```python
from build123d import *

# Parameters (mm, degrees)
F0_W     = 60
F0_H     = 20.115981
F0_R     = 3
F0_R_2   = 1.308767
F1_DEPTH = 10
F3_R     = 6
F4_W     = 7.989561
F4_H     = 2.429715
F5_DEPTH = 10


with BuildPart() as f1:
    # F0 (on Front) → F1 (new body)
    with BuildSketch(Plane.XZ):
        with Locations((30, 10.05799)):
            Rectangle(F0_W, F0_H)
        with Locations((6.314433, 11.456186)):
            Circle(F0_R, mode=Mode.SUBTRACT)
        with Locations((26.120204, 12.682377)):
            Circle(F0_R_2, mode=Mode.SUBTRACT)
        with Locations((50, 11.406668)):
            Circle(F0_R, mode=Mode.SUBTRACT)
    extrude(amount=F1_DEPTH)

    # F3
    f3_edges = [f1.edges().sort_by_distance(p)[0] for p in [
        (0, -5, 0),
        (0, -5, 20.115981),
        (60, -5, 0),
        (60, -5, 20.115981),
    ]]
    fillet(f3_edges, radius=F3_R)

    # F4 (on face) → F5 (cut)
    with BuildSketch(Plane.XY.offset(20.115981)):
        with Locations((24.271051, -1.214857)):
            Rectangle(F4_W, F4_H)
    extrude(amount=-F5_DEPTH, mode=Mode.SUBTRACT)


solid = f1.part
```
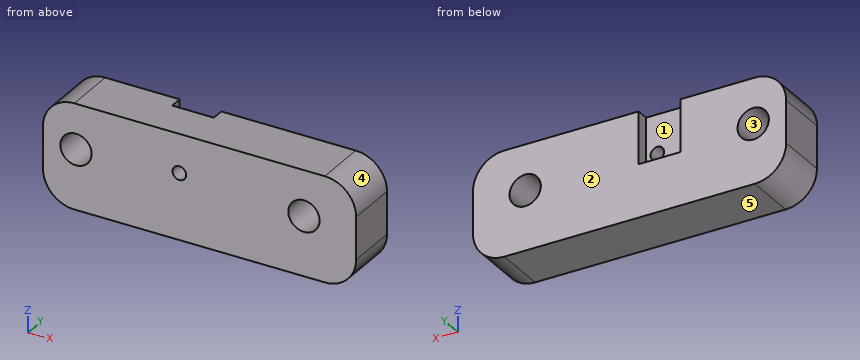
Model file for the job. Use its own axes, mm. Face numbers are marked on the shaded views. A direction names the side the tool comes from. Give positions to 0.01 mm unless a question says otherwise; leave off trailing zeros. Loops run counter-clockwise (first coordinate to the right, second up) from the corner with the lowest first, then second, coordinate; pieces in that order, holes last. Notation, with made-up numbers: (1.25, -13.5) -> (13.25, -13.5) arc R19 ccw to (13.25, 13.5) -> close; hole circle Ø9 at (28.5, 83). An arc over 180 degrees is marked (long way). Use CSV: the item, a comma, the result in double quotes. Start each with the question number.
1) Wall check: line 1 (Z direction, x = 50, y = -6.5); line 2 (X direction, y = -0.75, z = 9); line 3 (X direction, y = -6.25, z = 9.75). Give the ranges that are in metal, low to high.
2) Flat gauge pins, fed straight in: pin 1 Ø4 at (x, z) = (25.5, 15) entering from +Y; pin 2 Ø5.5 at (x, z) = (50, 11.41) entering from -Y; pin 3 Ø2.5 at (x, y) = (22.5, -0.5) entering from +Z; pin 4 Ø0.7 at (y, z) = (-1.5, 15.5) entering from +X. Where does each tip first touch, or does it go through?
3) Slice it at C-C on z = 18.5. Give the cut face in (x, y), plus the area to 3 significant figures.
4) Mould opens along X. For the marked faces 3, 4 and 5 say: released by +X, released by -X, zero draft, split by the parting line, or undercut.
5) Tool access for the marked faces 1 and 2: list every direction of +Z, -Z, +X, -X, +Y, -Y with a clear straight run to the whole face (end or side of a thin tool).
6) Slice it at B-B on y = -0.75. Give the cut face in (x, z).
7) Slice it at A-A on x = 50. Give the cut face in (y, z).
8) Slice it at D-D on y = -8. Give the cut face in (x, z).
Computed values:
1,line 1,"z = 0 to 8.41, 14.41 to 20.12"
1,line 2,"x = 0 to 4.59, 8.04 to 48.21, 51.79 to 60"
1,line 3,"x = 0 to 3.85, 8.78 to 47.5, 52.5 to 60"
2,pin 1,"stops at y = -2.43"
2,pin 2,"passes through"
2,pin 3,"stops at z = 10.12"
2,pin 4,"stops at x = 59.91"
3,outline,"(1.9, -10) -> (58.1, -10) -> (58.1, 0) -> (28.27, 0) -> (28.27, -2.43) -> (20.28, -2.43) -> (20.28, 0) -> (1.9, 0) -> close"
3,area,"543 mm^2"
4,face 3,"undercut"
4,face 4,"released by +X"
4,face 5,"zero draft"
5,face 1,"+Z, +Y"
5,face 2,"+Z, -Z, +X, -X, +Y"
6,outline,"(0, 6) arc R6 ccw to (6, 0) -> (54, 0) arc R6 ccw to (60, 6) -> (60, 14.12) arc R6 ccw to (54, 20.12) -> (28.27, 20.12) -> (28.27, 10.12) -> (20.28, 10.12) -> (20.28, 20.12) -> (6, 20.12) arc R6 ccw to (0, 14.12) -> close; hole circle Ø6 at (6.31, 11.46); hole circle Ø6 at (50, 11.41)"
7,outline,"(-10, 0) -> (0, 0) -> (0, 8.41) -> (-10, 8.41) -> close; (-10, 14.41) -> (0, 14.41) -> (0, 20.12) -> (-10, 20.12) -> close"
8,outline,"(0, 6) arc R6 ccw to (6, 0) -> (54, 0) arc R6 ccw to (60, 6) -> (60, 14.12) arc R6 ccw to (54, 20.12) -> (6, 20.12) arc R6 ccw to (0, 14.12) -> close; hole circle Ø6 at (6.31, 11.46); hole circle Ø2.62 at (26.12, 12.68); hole circle Ø6 at (50, 11.41)"
